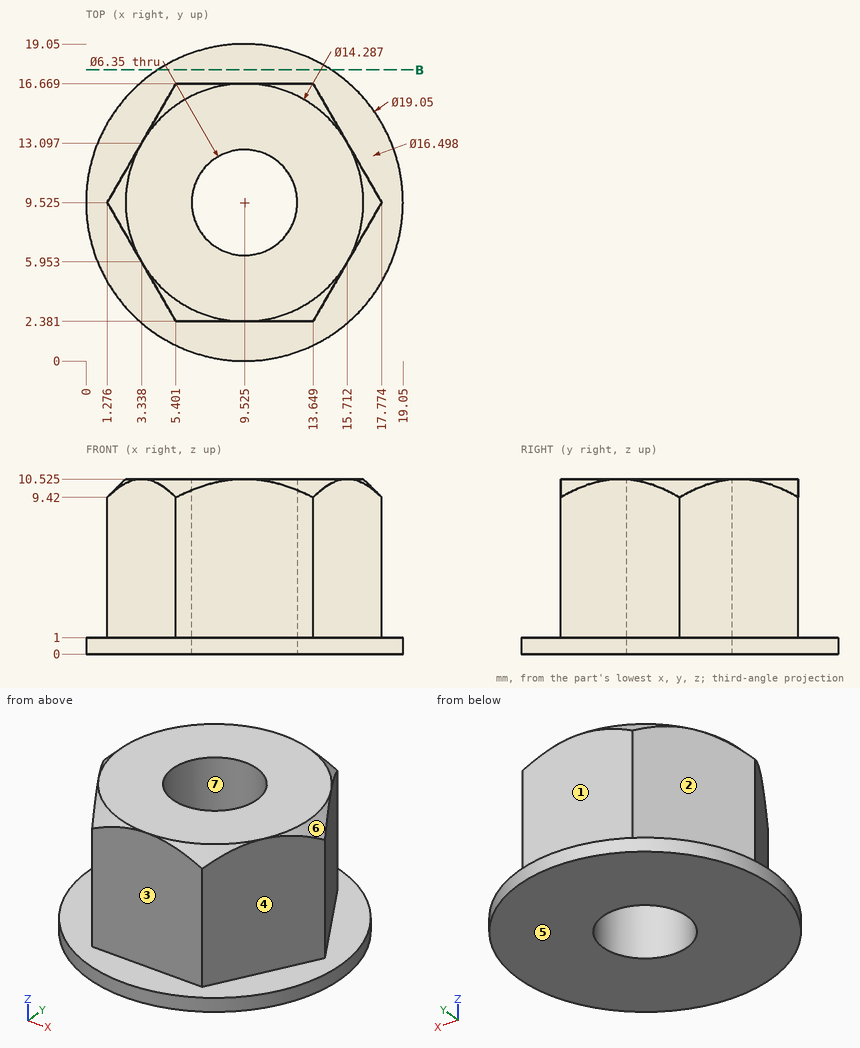
Part print with two shaded views. Sizes in mm from the minimum x, y, z corner. A direction names the side the tool comes from. Round coordinates to 2 decimals unless told otherwise and drop trailing zeros. Order: outer loops, then holes, each group sorted by start corner. A loop starts at its lowest first (then second) coordinate and runs counter-clockwise, first axis right, second up. Notation, with made-up numbers: M -17,67.5 L 2,67.5 A25 cw 2,98.5 Z; hole C -33.5,43.5 d2. An arc over 180 degrees is marked long. Use CSV: the item, a comma, the result in double quotes. Start each with the question number.
(1) Flat gauge pins, fed straight in: P1, Ø5, axis at x = 11, z = 7.5, coming from the -Y side; P2, Ø4, axis at x = 8, z = 7.5, coming from the +Y side; P3, Ø3, axis at y = 10.5, z = 6.5, coming from the +X side. Where does each tip first touch, or does it go through?
(2) Tool access for the marked faces 1, 2, 3 and 4: list every direction of +Z, -Z, +X, -X, +Y, -Y with a clear straight run to the whole face (end or side of a thin tool).
(3) Cut at B-B on y = 17.5. List the corners of the cut face in (x, z).
(4) Mould opens along X. For the marked faces 5, 6 and 7 say: +X half, -X half, draft (parallel to the pull), parting line (faces both ways), or undercut.
(5) Drill centre lines: probe 1 along Y at (x, z) = (7, 6); probe 2 along Y at (x, z) = (13, 6.25); probe 3 along Y at (x, z) = (6.75, 9.25) (1 decimal). Where is each one in solid material? Low to high.
Findings:
1,P1,"stops at y = 2.38"
1,P2,"stops at y = 16.67"
1,P3,"stops at x = 17.77"
2,face 1,"+Z, +X, -X, +Y"
2,face 2,"+Z, -X, +Y"
2,face 3,"+Z, +X, -X, -Y"
2,face 4,"+Z, +X, -Y"
3,outline,"M 4.32,0 L 14.73,0 L 14.73,1 L 4.32,1 Z"
4,face 5,"draft"
4,face 6,"+X half"
4,face 7,"undercut"
5,probe 1,"y = 2.38 to 7.6, 11.45 to 16.67"
5,probe 2,"y = 2.38 to 16.67"
5,probe 3,"y = 2.4 to 8, 11.1 to 16.7"
